Answer from the drawing. Dimensions are ordinates in mm from the lowest x, y and z of the part. Give positions to 0.01 mm unless a question says otherwise; leave off trailing zeros. Order: outer loops, then holes, each group sorted by start corner. A loop starts at its lowest first (then second) coordinate and runs counter-clockwise, first axis right, second up. Notation, with made-up numbers: (-38, 65) - (-22, 65) arc R3 cw to (-22, 69) - close; hole circle Ø11 at (47, 16). An arc over 180 degrees is marked (long way). Answer in a Markdown table with one row per item.
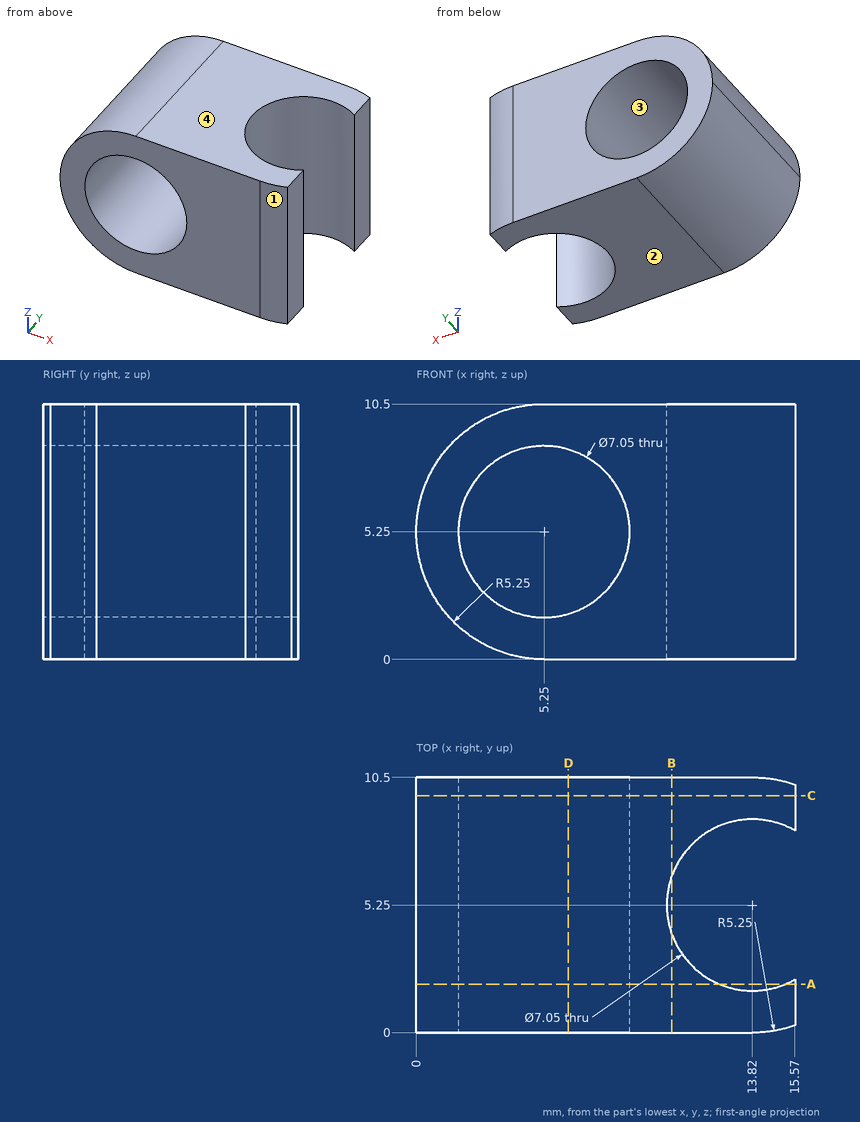
Item 1: Each of these flat-tipped pins is pushed along its axis until it touches: P1, Ø2, axis at x = 1.5, z = 9.5, coming from the +Y side; P2, Ø1.5, axis at x = 2, y = 6.5, coming from the +Z side; P3, Ø1, axis at y = 4, z = 1.5, coming from the -X side. Where does it stop, or does it pass through?
Answer block:
| item | result |
|---|---|
| P1 | y = 10.5 |
| P2 | z = 9.87 |
| P3 | x = 1.13 |
Item 2: Find section B-B on x = 10.5. Write down the section's boundary in (y, z).
Answer block:
| item | result |
|---|---|
| outline | (0, 0) - (4.07, 0) - (4.07, 10.5) - (0, 10.5) - close; (6.43, 0) - (10.5, 0) - (10.5, 10.5) - (6.43, 10.5) - close |
Item 3: Find section D-D on x = 6.25. Write down the section's boundary in (y, z), then the cut area to 3 significant figures.
Answer block:
| item | result |
|---|---|
| outline | (0, 0) - (10.5, 0) - (10.5, 1.87) - (0, 1.87) - close; (0, 8.63) - (10.5, 8.63) - (10.5, 10.5) - (0, 10.5) - close |
| area | 39.3 mm² |
Item 4: Find section C-C on y = 9.75. Write down the section's boundary in (x, z) (3 decimals), then the cut area to 3 significant figures.
Answer block:
| item | result |
|---|---|
| outline | (0, 5.25) arc R5.25 ccw to (5.25, 0) - (15.57, 0) - (15.57, 10.5) - (5.25, 10.5) arc R5.25 ccw to start; hole circle Ø7.05 at (5.25, 5.25) |
| area | 113 mm² |
Item 5: Consider line 1 (Y direction, x = 13.75, z = 6); line 2 (Z direction, x = 3.5, y = 8.5); line 3 (X direction, y = 2.75, z = 6.25) (3 decimals). Determine where each line is inside the solid, lowest interval first.
Answer block:
| item | result |
|---|---|
| line 1 | 0 to 1.73, 8.77 to 10.5 |
| line 2 | 0.3 to 2.19, 8.31 to 10.2 |
| line 3 | 0.096 to 1.87, 8.63 to 11.335 |
Item 6: Find section A-A on y = 2. Write down the section's boundary in (x, z) (3 decimals).
Answer block:
| item | result |
|---|---|
| outline | (0, 5.25) arc R5.25 ccw to (5.25, 0) - (12.455, 0) - (12.455, 10.5) - (5.25, 10.5) arc R5.25 ccw to start; (15.185, 0) - (15.57, 0) - (15.57, 10.5) - (15.185, 10.5) - close; hole circle Ø7.05 at (5.25, 5.25) |
Item 7: Determine the mould class of the marked faces 1, 2, 3 and 4 for opening direction Z: pulls with the +Z half, pulls with the -Z half, needs draft (parallel to the pull), parting line crosses it, or undercut.
Answer block:
| item | result |
|---|---|
| face 1 | needs draft |
| face 2 | pulls with the -Z half |
| face 3 | undercut |
| face 4 | pulls with the +Z half |
